from build123d import *

# Parameters (mm, degrees)
EXTRUDE_1_DEPTH     = 13
CUT_EXTRUDE_1_DEPTH = 49.78979572841993
CUT_EXTRUDE_2_DEPTH = 72.67669327248296
FILLET_1_R          = 2
CUT_EXTRUDE_3_DEPTH = 13
SKETCH_8_R          = 2.000000000000001
SKETCH_8_R_2        = 2.0000000000000018
CUT_EXTRUDE_4_DEPTH = 13
CUT_EXTRUDE_5_DEPTH = 6
SKETCH_10_R         = 3
SKETCH_10_R_2       = 3.0000000000000013
EXTRUDE_2_DEPTH     = 4
CUT_EXTRUDE_6_REACH = 75.821
SKETCH_11_R         = 1.7500000000000004
SKETCH_11_R_2       = 1.7499999999999998


with BuildPart() as part:
    # 草圖4 → 填料-伸長1 (new body)
    with BuildSketch(Plane(origin=(0, 0, 0), x_dir=(0, 0, -1), z_dir=(1, 0, 0))):
        Polygon((0, 0), (-60, -7.35e-15), (-60, 4.999999999999993), (-19.982621227151128, 36.9938962327247), (6e-16, 12), align=None)
    extrude(amount=EXTRUDE_1_DEPTH)

    # 草圖5 → 除料-伸長1 (cut, through all)
    with BuildSketch(Plane(origin=(0, 32.31453899318016, 25.83547546241596), x_dir=(1, 0, 0), z_dir=(0, 0.7810592572726445, 0.6244569133484753))):
        Polygon((0, 3.4934829601818222), (5, 3.4934829601818222), (5.000000000000004, -49.04518650741456), (0, -49.04518650741456), align=None)
    extrude(amount=-CUT_EXTRUDE_1_DEPTH, mode=Mode.SUBTRACT)

    # 草圖6 → 除料-伸長2 (cut, through all)
    with BuildSketch(Plane(origin=(13, 0, 0), x_dir=(0, 0, -1), z_dir=(1, 0, 0))):
        Polygon((-24.98262122715113, 27.87514563803557), (-24.982621227151125, 3.9999999999999933), (-54.84521562029527, 3.99999999999999), align=None)
        Polygon((-16.982621227151128, 26.835985196390023), (-1.9496281407001657, 8.032993086450977), (-5.982621227151128, 3.9999999999999964), (-16.982621227151128, 3.9999999999999942), align=None)
    extrude(amount=-CUT_EXTRUDE_2_DEPTH, mode=Mode.SUBTRACT)

    # 圓角1
    fillet_1_edges = [part.edges().sort_by_distance(p)[0] for p in [
        (9.000000000000002, 3.99999999999999, 54.84521562029527),
        (9, 27.87514563803557, 24.98262122715113),
        (9, 3.9999999999999933, 24.982621227151125),
        (9, 26.835985196390023, 16.982621227151128),
        (9, 3.9999999999999964, 5.982621227151128),
        (9, 3.9999999999999942, 16.982621227151128),
        (9, 8.032993086450977, 1.9496281407001657),
    ]]
    fillet(fillet_1_edges, radius=FILLET_1_R)

    # 草圖7 → 除料-伸長3 (cut)
    with BuildSketch(Plane(origin=(0, 2.181529586150628, -2.728617206174244), x_dir=(1, 0, 0), z_dir=(0, -0.6244569133484752, 0.7810592572726445))):
        Polygon((0, 9.372711087271734), (4.999999999999999, 9.372711087271734), (4.999999999999999, 4.369584430641977), (0, 4.369584430641976), align=None)
    extrude(amount=-CUT_EXTRUDE_3_DEPTH, mode=Mode.SUBTRACT)

    # 草圖8 → 除料-伸長4 (cut)
    with BuildSketch(Plane(origin=(0, 4.679357239544419, -5.852854235264727), x_dir=(-1, 0, 0), z_dir=(0, 0.6244569133484724, -0.7810592572726467))):
        with Locations(Location((-4, 34.372711087271774, 0), (0, 0, 90))):
            Circle(SKETCH_8_R)
        with Locations(Location((-4, 16.372711087271757, 0), (0, 0, 90))):
            Circle(SKETCH_8_R_2)
    extrude(amount=-CUT_EXTRUDE_4_DEPTH, mode=Mode.SUBTRACT)

    # 草圖9 → 除料-伸長5 (cut)
    with BuildSketch(Plane.ZY.offset(-5)):
        with BuildLine():
            Line((20.609030602847792, 31.371831550240223), (3.0671165568141214, 9.430727107234867))
            ThreePointArc((3.0671165568141214, 9.430727107234867), (2.632312431238594, 8.07090805355147), (3.215021508986313, 6.767599718164824))
            Line((3.215021508986313, 6.767599718164824), (5.396834789524223, 4.585786437626903))
            ThreePointArc((5.396834789524223, 4.585786437626903), (6.04568148716714, 4.1522409349774225), (6.811048351897321, 3.9999999999999956))
            Line((6.811048351897321, 3.9999999999999956), (49.14086927004922, 3.9999999999999907))
            ThreePointArc((49.14086927004922, 3.9999999999999907), (51.02822681819565, 5.338273859172296), (50.38978309674617, 7.56211851454527))
            Line((50.38978309674617, 7.56211851454527), (20.609030602847792, 31.371831550240223))
        make_face()
    extrude(amount=-CUT_EXTRUDE_5_DEPTH, mode=Mode.SUBTRACT)

    # 草圖10 → 填料-伸長2 (add)
    with BuildSketch(Plane.XZ):
        with Locations((9.999999999999998, 55)):
            Circle(SKETCH_10_R)
        with Locations((9.999999999999998, 5)):
            Circle(SKETCH_10_R_2)
    extrude(amount=EXTRUDE_2_DEPTH)

    # 草圖11 → 除料-伸長6 (cut, up to next)
    with BuildSketch(Plane(origin=(0, -4, -4.9e-16), x_dir=(-1, 0, 0), z_dir=(0, -1, -1.2e-16)), mode=Mode.PRIVATE) as cut_extrude_6_sk1:
        with Locations(Location((-9.999999999999998, -55, 0), (0, 0, 90))):
            Circle(SKETCH_11_R)
    cut_extrude_6_tool1 = extrude(cut_extrude_6_sk1.sketch, amount=-CUT_EXTRUDE_6_REACH, mode=Mode.PRIVATE) & part.part
    # 草圖11 → 除料-伸長6 (cut, up to next)
    with BuildSketch(Plane(origin=(0, -4, -4.9e-16), x_dir=(-1, 0, 0), z_dir=(0, -1, -1.2e-16)), mode=Mode.PRIVATE) as cut_extrude_6_sk2:
        with Locations(Location((-9.999999999999998, -5, 0), (0, 0, 90))):
            Circle(SKETCH_11_R_2)
    cut_extrude_6_tool2 = extrude(cut_extrude_6_sk2.sketch, amount=-CUT_EXTRUDE_6_REACH, mode=Mode.PRIVATE) & part.part
    add(cut_extrude_6_tool1.solids().sort_by_distance((10, -4, 55))[0], mode=Mode.SUBTRACT)
    add(cut_extrude_6_tool2.solids().sort_by_distance((10, -4, 5))[0], mode=Mode.SUBTRACT)


solid = part.part
Read the model definition and answer for the solid it produces. Units are mm, in the model's axes. A direction names the side the tool comes from. Give positions to 0.01 mm unless a question says otherwise; leave off trailing zeros. Write each loop counter-clockwise with the first axis right and the second up, starting at its lowest first coordinate (ties: lowest second). Pieces come first, ordered by that corner, then holes. Notation, with made-up numbers: (73.25, -28) - (106.25, -28) arc R21 ccw to (106.25, -23) - close; hole circle Ø10 at (34, 33.5). An arc over 180 degrees is marked (long way). Use CSV: the item, a comma, the result in double quotes. Start each with the question number.
Item 1: The part is cut by section D-D, the plane y = 14.5. Count the separate pieces of the cut face and the enclosed holes in it, and give its area (3 significant figures).
Item 2: The mould has two halves that part along Z. Classify faces 6 (the flat face through (6.41, 24.67, 10.13)), 7 (the flat face through (11, 18, 21)), 8 (the flat face through (0, 23, 11)): pulls with the +Z half, pulls with the -Z half, needs draft (parallel to the pull), parting line crosses it, or undercut.
Item 3: The part is cut by section A-A, the plane x = 10. Give the vertices of the cut face in (y, z).
Item 4: For faces 1 (the cylindrical face through (10, -2, 58)), 2 (the flat face through (13, 12, 23)), 3 (the flat face through (8.17, 5.69, 4.29)), 4 (the flat face through (6.41, 22.14, 13.23)), 5 (the flat face through (2.465, 10.734, 1.584)), determine the directions among +Z, -Z, +X, -X, +Y, -Y from which every point of the face is accessible in a straight line to the end or side of a thin tool.
Item 5: Consider line 1 (Z direction, x = 10, y = 0.5); line 2 (X direction, y = 1.5, z = 5); line 3 (Z direction, x = 10, y = -0.25). Determine where each line is inside the solid, lowest interval first.
Item 6: The part is cut by section B-B, the plane x = 2.75. Give the vertices of the cut face in (y, z).
Item 7: Flat-ended cylindrical pins translate along their axes: P1, Ø6.5, axis at x = 7, z = 37, coming from the +Y side; P2, Ø1, axis at x = 11, y = 24, coming from the -Z side; P3, Ø1, axis at x = 10, z = 35.5, coming from the -Y side. Find the tip coordinate at first contact, or state that the pin passes through.
Item 8: The part is cut by section C-C, the plane z = 39. Give the vertices of the cut face in (x, y), and give its area (3 significant figures).
Taken from the geometry:
1,separate pieces,"3"
1,enclosed holes,"0"
1,area,"128 mm2"
2,face 6,"pulls with the -Z half"
2,face 7,"undercut"
2,face 8,"needs draft"
3,outline,"(-4, 2) - (0, 2) - (0, 0) - (12, 0) - (36.99, 19.98) - (10.4, 53.25) - (-4, 53.25) - (-4, 52) - (0, 52) - (0, 8) - (-4, 8) - (-4, 6.75) - (4, 6.75) arc R2 cw to (4, 6.81) - (4, 49.14) arc R2 cw to (7.56, 50.39) - (31.37, 20.61) - (9.43, 3.07) arc R2 cw to (6.77, 3.22) - (6.73, 3.25) - (-4, 3.25) - close; (-4, 56.75) - (7.6, 56.75) - (5, 60) - (0, 60) - (0, 58) - (-4, 58) - close"
4,face 1,"-Y"
4,face 2,"+Z, -Z, +X, +Y, -Y"
4,face 3,"+X, -X"
4,face 4,"-X"
4,face 5,"-Z, -X, -Y"
5,line 1,"0 to 3.25, 6.75 to 53.25, 56.75 to 60"
5,line 2,"5 to 8.25, 11.75 to 13"
5,line 3,"2 to 3.25, 6.75 to 8, 52 to 53.25, 56.75 to 58"
6,outline,"(9.5, 3.12) - (12, 0) - (16.25, 3.4) - (13.75, 6.52) - close; (16.19, 8.47) - (18.69, 5.35) - (30.31, 14.64) - (27.81, 17.76) - close; (30.25, 19.71) - (32.75, 16.59) - (36.99, 19.98) - (34.5, 23.11) - close"
7,P1,"y = 25.99"
7,P2,"z = 9.19"
7,P3,"y = 0"
8,outline,"(5, 0) - (13, 0) - (13, 4) - (5, 4) - close; (5, 16.67) - (13, 16.67) - (13, 21.79) - (5, 21.79) - close"
8,area,"73.0 mm2"
